Autodesk Inventor part; units mm, degrees
ref_plane "YZ Plane" through (0, 0, 0) normal (1, 0, 0) x (0, 1, 0)
ref_plane "XZ Plane" through (0, 0, 0) normal (0, 1, 0) x (-1, 0, 0)
ref_plane "XY Plane" through (0, 0, 0) normal (0, 0, 1) x (1, 0, 0)
sketch "スケッチ1" plane through (0, 0, 0) normal (0, 0, 1) x (1, 0, 0)
  line L0 (-10, -10) -> (10, -10)
  line L1 (10, -10) -> (10, 10)
  line L2 (10, 10) -> (-10, 10)
  line L3 (-10, 10) -> (-10, -10)
  line L4 (-10, -10) -> (10, 10) construction
  line L5 (10, -10) -> (-10, 10) construction
  line L6 (9, -9) -> (-9, -9)
  line L7 (-9, -9) -> (-9, 9)
  line L8 (-9, 9) -> (9, 9)
  line L9 (9, 9) -> (9, -9)
  line L10 (9, -9) -> (-9, 9) construction
  line L11 (-9, -9) -> (9, 9) construction
  line L12 (9, 9) -> (10, 9)
  line L13 (9, -9) -> (10, -9)
  point P0 (0, 0)
  dimension "d0" = 20
  dimension "d1" = 20
  dimension "d2" = 1
extrude "押し出し1" add sketch "スケッチ1" along normal blind 250 contours L3 L2 L1 L12 L8 L7 L6 L13 L0
sketch "スケッチ2" plane through (-10, -10, 0) normal (0, -1, 0) x (1, 0, 0)
  circle A0 centre (10, 155) radius 1.75
  circle A1 centre (10, 125) radius 1.75
  line L0 (0, 0) -> (0, 250)
  line L1 (0, 250) -> (20, 250)
  point P0 (10, 0)
  dimension "d5" = 3.5
  dimension "d7" = 10
  dimension "d8" = 95
  dimension "d9" = 30
extrude "押し出し2" cut sketch "スケッチ2" against normal up to surface (1 mm away)
sketch "スケッチ3" plane through (-9, -9, 0) normal (1, 0, 0) x (0, 0, -1)
  line L0 (-156.75, 0) -> (-153.25, 0)
  circle A0 centre (-170, 9) radius 2.25
  circle A1 centre (-140, 9) radius 2.25
  line L1 (0, -1) -> (-250, -1)
  point P0 (0, 9)
  point P1 (-155, 0)
  dimension "d12" = 4.5
  dimension "d13" = 4.5
  dimension "d14" = 15
  dimension "d15" = 10
  dimension "d16" = 30
extrude "押し出し3" cut sketch "スケッチ3" against normal through all
sketch "スケッチ5" plane through (-10, 10, 0) normal (0, 1, 0) x (1, 0, 0)
  circle A0 centre (10, -240) radius 1.75
  circle A1 centre (10, -10) radius 1.75
  circle A2 centre (10, -25) radius 1.75
  circle A3 centre (10, -230) radius 1.75
  circle A4 centre (10, -40) radius 1.75
  line L0 (20, 0) -> (0, 0)
  line L1 (20, -250) -> (0, -250)
  point P0 (10, 0)
  point P1 (10, 0)
  dimension "d19" = 3.5
  dimension "d20" = 10
  dimension "d21" = 10
  dimension "d22" = 10
  dimension "d23" = 15
  dimension "d24" = 15
extrude "押し出し4" cut sketch "スケッチ5" against normal through all
sketch "スケッチ6" plane through (-10, 10, 0) normal (0, 1, 0) x (1, 0, 0)
  circle A0 centre (10, -210) radius 1.75
  circle A1 centre (10, -190) radius 1.75
  circle A2 centre (10, -240) radius 1.75
  line L0 (20, -250) -> (0, -250)
  point P0 (10, 0)
  dimension "d27" = 40
  dimension "d28" = 20
extrude "押し出し5" cut sketch "スケッチ6" against normal through all contours A0 | A1
equation "\"d24\" = d23"
properties part number "gear_plate_pole" material "アルミニウム 6061"
Could you check a few things on this model? Use its own coordinates, in mm. A direction names the side the tool comes from. Give positions to 0.01 mm unless a question says otherwise; leave off trailing zeros. Loops run counter-clockwise (first coordinate to the right, second up) from the corner with the lowest first, then second, coordinate; pieces in that order, holes last. Notation, with made-up numbers: (64.5, 29) -> (123.5, 29) arc R22 ccw to (123.5, 44) -> close; hole circle Ø11 at (-39.75, 81.5). An arc over 180 degrees is marked (long way). Return JSON: item names as keys, results as strings.
Item 1: If we section it at C-C on z = 206: List the corners of the cut face in (x, y) for me, plus the area to 3 significant figures.
Geometry results:
{"outline": "(-10, -10) -> (10, -10) -> (10, -9) -> (-9, -9) -> (-9, 9) -> (10, 9) -> (10, 10) -> (-10, 10) -> close", "area": "58.0 mm²"}
Item 2: Which directions (+Z, -Z, +X, -X, +Y, -Y) give clear straight access to the entire face, cutting with the end or side of a thin tool? Please do faces 5 (the flat face through (1, -9, 123)), 6 (the flat face through (-9.7, 0, 0)).
Geometry results:
{"face 5": "+Z, -Z, +X", "face 6": "-Z, +X, -X, +Y, -Y"}
Item 3: I need wall thicknesses on L1, parallel to Y at x = 9, z = 94; L2, parallel to X at y = 9.5, z = 25; L3, parallel to X at y = -6, z = 239. Which ranges of each line are inside material? Lowest first, please. Write a range as from..to.
Geometry results:
{"L1": "y = -10..-9, 9..10", "L2": "x = -10..-1.75, 1.75..10", "L3": "x = -10..-9"}
Item 4: If we section it at A-A on z = 170: List the corners of the cut face in (x, y) for me, plus the area to 3 significant figures.
Geometry results:
{"outline": "(-10, -10) -> (10, -10) -> (10, -9) -> (-9, -9) -> (-9, -2.25) -> (-10, -2.25) -> close; (-10, 2.25) -> (-9, 2.25) -> (-9, 9) -> (10, 9) -> (10, 10) -> (-10, 10) -> close", "area": "53.5 mm²"}
Item 5: If we section it at B-B on y = 0: List the corners of the cut face in (x, z) for me.
Geometry results:
{"outline": "(-10, 0) -> (-9, 0) -> (-9, 137.75) -> (-10, 137.75) -> close; (-10, 142.25) -> (-9, 142.25) -> (-9, 167.75) -> (-10, 167.75) -> close; (-10, 172.25) -> (-9, 172.25) -> (-9, 250) -> (-10, 250) -> close"}
Item 6: We'd pull the mould along Y, two halves only. Please class faces 1 (the flat face through (-9, 0, 123)), 2 (the flat face through (-10, 0, 123)), 3 (the flat face through (0, 10, 123)), 4 (the flat face through (0, -10, 123)): +Y half, -Y half, draft (parallel to the pull), parting line (faces both ways), or undercut.
Geometry results:
{"face 1": "undercut", "face 2": "draft", "face 3": "+Y half", "face 4": "-Y half"}
Item 7: I'm going to push flat-ended pins straight in: pin 1 (3 mm diameter, centred on y = -5.5, z = 204, fed in from +X); pin 2 (3 mm diameter, centred on x = 0, z = 155, fed in from -Y). Where does each tip first touch, or does it pass through?
Geometry results:
{"pin 1": "stops at x = -9", "pin 2": "stops at y = 9"}
